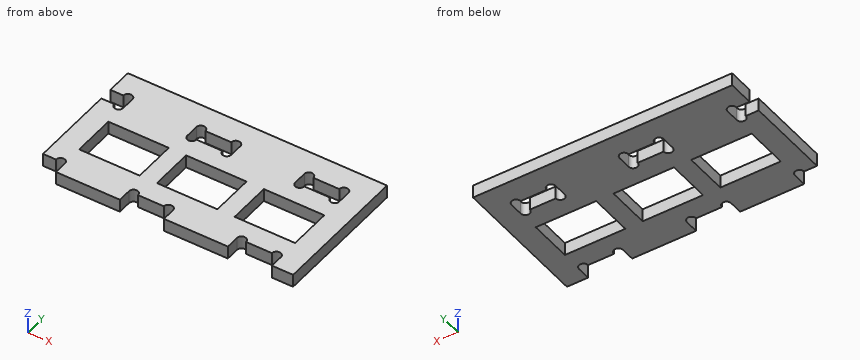
from build123d import *

# Parameters (mm, degrees)
SKETCH_1_W          = 14
SKETCH_1_H          = 10
EXTRUDE_1_DEPTH     = 3
SKETCH_2_W          = 10
SKETCH_2_H          = 32.2
CUT_EXTRUDE_1_DEPTH = 10


with BuildPart() as part:
    # 草图1 → 凸台-拉伸1 (new body)
    with BuildSketch(Plane.XY):
        with BuildLine():
            Line((-19.9, -16.1), (-5.1, -16.1))
            Line((-5.1, -16.1), (-5.1, -13))
            ThreePointArc((-5.1, -13), (-4.05, -11.95), (-3, -13))
            Line((-3, -13), (3, -13))
            ThreePointArc((3, -13), (4.05, -11.95), (5.1, -13))
            Line((5.1, -13), (5.1, -16.1))
            Line((5.1, -16.1), (19.9, -16.1))
            Line((19.9, -16.1), (19.9, -13))
            ThreePointArc((19.9, -13), (20.95, -11.95), (22, -13))
            Line((22, -13), (28, -13))
            ThreePointArc((28, -13), (29.05, -11.95), (30.1, -13))
            Line((30.1, -13), (30.1, -16.1))
            Line((30.1, -16.1), (35, -16.1))
            Line((35, -16.1), (35, 16.1))
            Line((35, 16.1), (-35, 16.1))
            Line((-35, 16.1), (-35, -16.1))
            Line((-35, -16.1), (-30.1, -16.1))
            Line((-30.1, -16.1), (-30.1, -13))
            ThreePointArc((-30.1, -13), (-29.05, -11.95), (-28, -13))
            Line((-28, -13), (-22, -13))
            ThreePointArc((-22, -13), (-20.95, -11.95), (-19.9, -13))
            Line((-19.9, -13), (-19.9, -16.1))
        make_face()
        with Locations((-13, -3)):
            Rectangle(SKETCH_1_W, SKETCH_1_H, mode=Mode.SUBTRACT)
        with Locations((5, -3)):
            Rectangle(SKETCH_1_W, SKETCH_1_H, mode=Mode.SUBTRACT)
        with Locations((23, -3)):
            Rectangle(SKETCH_1_W, SKETCH_1_H, mode=Mode.SUBTRACT)
        with BuildLine():
            Line((-22, 7), (-28, 7))
            ThreePointArc((-28, 7), (-29.05, 5.95), (-30.1, 7))
            Line((-30.1, 7), (-30.1, 10.1))
            ThreePointArc((-30.1, 10.1), (-29.05, 11.15), (-28, 10.1))
            Line((-28, 10.1), (-22, 10.1))
            ThreePointArc((-22, 10.1), (-20.95, 11.15), (-19.9, 10.1))
            Line((-19.9, 10.1), (-19.9, 7))
            ThreePointArc((-19.9, 7), (-20.95, 5.95), (-22, 7))
        make_face(mode=Mode.SUBTRACT)
        with BuildLine():
            Line((3, 7), (-3, 7))
            ThreePointArc((-3, 7), (-4.05, 5.95), (-5.1, 7))
            Line((-5.1, 7), (-5.1, 10.1))
            ThreePointArc((-5.1, 10.1), (-4.05, 11.15), (-3, 10.1))
            Line((-3, 10.1), (3, 10.1))
            ThreePointArc((3, 10.1), (4.05, 11.15), (5.1, 10.1))
            Line((5.1, 10.1), (5.1, 7))
            ThreePointArc((5.1, 7), (4.05, 5.95), (3, 7))
        make_face(mode=Mode.SUBTRACT)
        with BuildLine():
            Line((30.1, 10.1), (30.1, 7))
            ThreePointArc((30.1, 7), (29.05, 5.95), (28, 7))
            Line((28, 7), (22, 7))
            ThreePointArc((22, 7), (20.95, 5.95), (19.9, 7))
            Line((19.9, 7), (19.9, 10.1))
            ThreePointArc((19.9, 10.1), (20.95, 11.15), (22, 10.1))
            Line((22, 10.1), (28, 10.1))
            ThreePointArc((28, 10.1), (29.05, 11.15), (30.1, 10.1))
        make_face(mode=Mode.SUBTRACT)
    extrude(amount=EXTRUDE_1_DEPTH)

    # 草图2 → 切除-拉伸1 (cut)
    with BuildSketch(Plane.XY.offset(3)):
        with Locations((-30, 0)):
            Rectangle(SKETCH_2_W, SKETCH_2_H)
    extrude(amount=-CUT_EXTRUDE_1_DEPTH, mode=Mode.SUBTRACT)


solid = part.part
Verification items for the finished model (mm, model axes). Coordinates: 2 decimals unless noted, no trailing zeros. Order: outer loops, then holes, each group sorted by start corner. A loop starts at its lowest first (then second) coordinate and runs counter-clockwise, first axis right, second up.
1. Scan lines: line 1 (X direction, y = -14, z = 0.65); line 2 (Y direction, x = 22.5, z = 0.95); line 3 (X direction, y = -4, z = 2.2). Record each from-to range of solid material in increasing order.
Results found:
line 1: x = -19.9 to -5.1, 5.1 to 19.9, 30.1 to 35
line 2: y = -13 to -8, 2 to 7, 10.1 to 16.1
line 3: x = -25 to -20, -6 to -2, 12 to 16, 30 to 35
2. Sectioned sample at C-C, the plane x = 26. Record the cut outline in (y, z).
Results found:
outline: (-13, 0) - (-8, 0) - (-8, 3) - (-13, 3) - close; (2, 0) - (7, 0) - (7, 3) - (2, 3) - close; (10.1, 0) - (16.1, 0) - (16.1, 3) - (10.1, 3) - close
3. Sectioned sample at A-A, the plane x = -20.95. Record the cut outline in (y, z), and give its area (4 significant figures).
Results found:
outline: (-11.95, 0) - (5.95, 0) - (5.95, 3) - (-11.95, 3) - close; (11.15, 0) - (16.1, 0) - (16.1, 3) - (11.15, 3) - close
area: 68.55 mm2
4. Go/stop test with flat-tipped pins: pin 1 Ø0.9 at (y, z) = (-14, 1) entering from -X; pin 2 Ø1.5 at (x, z) = (25, 1) entering from -Y. Record where each tip stops, or that it passes through.
Results found:
pin 1: stops at x = -19.9
pin 2: stops at y = -13
5. Sectioned sample at B-B, the plane y = 9. Record the cut outline in (x, z), and give its area (4 significant figures).
Results found:
outline: (-19.9, 0) - (-5.1, 0) - (-5.1, 3) - (-19.9, 3) - close; (5.1, 0) - (19.9, 0) - (19.9, 3) - (5.1, 3) - close; (30.1, 0) - (35, 0) - (35, 3) - (30.1, 3) - close
area: 103.5 mm2
6. Sectioned sample at D-D, the plane y = 0. Record the cut outline in (x, z).
Results found:
outline: (-25, 0) - (-20, 0) - (-20, 3) - (-25, 3) - close; (-6, 0) - (-2, 0) - (-2, 3) - (-6, 3) - close; (12, 0) - (16, 0) - (16, 3) - (12, 3) - close; (30, 0) - (35, 0) - (35, 3) - (30, 3) - close
